Could you check a few things on this model? Use its own coordinates, in mm. A direction names the side the tool comes from. Give positions to 0.01 mm unless a question says otherwise; leave off trailing zeros. Write each loop counter-clockwise with the first axis right and the second up, starting at its lowest first coordinate (ties: lowest second). Pieces come first, ordered by that corner, then holes. Notation, with made-up numbers: M 83.25,86.5 L 106.25,86.5 A18 cw 106.25,94.5 Z; hole C 81,40 d4. An arc over 180 degrees is marked long. Answer as CSV lines item,"result". Start each with the question number.
from build123d import *

# Parameters (mm, degrees)
SKETCH1_R             = 9.525
BOSS_EXTRUDE1_DEPTH   = 3.0226
SKETCH2_W             = 5.6007
SKETCH2_H             = 19.05
CUT_EXTRUDE1_DEPTH    = 2.794
SKETCH3_W             = 19.05
SKETCH3_H             = 5.6007
CUT_EXTRUDE2_DEPTH    = 2.794
SKETCH4_W             = 3.67665
SKETCH4_H             = 19.05
CUT_EXTRUDE3_DEPTH    = 1.27
SKETCH5_W             = 19.05
SKETCH5_H             = 3.67665
CUT_EXTRUDE4_DEPTH    = 1.27
CHAMFER1_SIZE         = 1.74640875
CHAMFER1_SIZE2        = 1.008289562
CHAMFER1_PART_2_SIZE  = 1.74640875
CHAMFER1_PART_2_SIZE2 = 1.008289562
CHAMFER1_PART_3_SIZE  = 1.74640875
CHAMFER1_PART_3_SIZE2 = 1.008289562
CHAMFER1_PART_4_SIZE  = 1.74640875
CHAMFER1_PART_4_SIZE2 = 1.008289562
SKETCH6_W             = 5.880735
SKETCH6_H             = 6.905625
CUT_EXTRUDE5_DEPTH    = 2.794
SKETCH7_W             = 6.905625
SKETCH7_H             = 5.880735
CUT_EXTRUDE6_DEPTH    = 2.794


with BuildPart() as part:
    # Sketch1 → Boss-Extrude1 (new body, symmetric)
    with BuildSketch(Plane.XY):
        Circle(SKETCH1_R)
    extrude(amount=BOSS_EXTRUDE1_DEPTH, both=True)

    # Sketch2 → Cut-Extrude1 (cut)
    with BuildSketch(Plane.XY.offset(3.0226)):
        Rectangle(SKETCH2_W, SKETCH2_H)
    extrude(amount=-CUT_EXTRUDE1_DEPTH, mode=Mode.SUBTRACT)

    # Sketch3 → Cut-Extrude2 (cut)
    with BuildSketch(Plane(origin=(0, 0, -3.0226), x_dir=(-1, 0, 0), z_dir=(0, 0, -1))):
        Rectangle(SKETCH3_W, SKETCH3_H)
    extrude(amount=-CUT_EXTRUDE2_DEPTH, mode=Mode.SUBTRACT)

    # Sketch4 → Cut-Extrude3 (cut)
    with BuildSketch(Plane.XY.offset(3.0226)):
        with Locations((7.686675, 0)):
            Rectangle(SKETCH4_W, SKETCH4_H)
        with Locations((-7.686675, 0)):
            Rectangle(SKETCH4_W, SKETCH4_H)
    extrude(amount=-CUT_EXTRUDE3_DEPTH, mode=Mode.SUBTRACT)

    # Sketch5 → Cut-Extrude4 (cut)
    with BuildSketch(Plane(origin=(0, 0, -3.0226), x_dir=(-1, 0, 0), z_dir=(0, 0, -1))):
        with Locations((0, 7.686675)):
            Rectangle(SKETCH5_W, SKETCH5_H)
        with Locations((0, -7.686675)):
            Rectangle(SKETCH5_W, SKETCH5_H)
    extrude(amount=-CUT_EXTRUDE4_DEPTH, mode=Mode.SUBTRACT)

    # Chamfer1
    chamfer1_edges = [part.edges().sort_by_distance(p)[0] for p in [
        (0, 9.525, -1.7526),
    ]]
    chamfer1_side = [part.faces().sort_by_distance(p)[0] for p in [
        (0, 7.346425268, -1.7526),
    ]]
    chamfer(chamfer1_edges, length=CHAMFER1_SIZE, length2=CHAMFER1_SIZE2, reference=chamfer1_side[0])

    # Chamfer1 part 2
    chamfer1_part_2_edges = [part.edges().sort_by_distance(p)[0] for p in [
        (0, -9.525, -1.7526),
    ]]
    chamfer1_part_2_side = [part.faces().sort_by_distance(p)[0] for p in [
        (0, -7.346425268, -1.7526),
    ]]
    chamfer(chamfer1_part_2_edges, length=CHAMFER1_PART_2_SIZE, length2=CHAMFER1_PART_2_SIZE2, reference=chamfer1_part_2_side[0])

    # Chamfer1 part 3
    chamfer1_part_3_edges = [part.edges().sort_by_distance(p)[0] for p in [
        (8.556610274, -4.184500642, 1.7526),
    ]]
    chamfer1_part_3_side = [part.faces().sort_by_distance(p)[0] for p in [
        (7.346425268, 0, 1.7526),
    ]]
    chamfer(chamfer1_part_3_edges, length=CHAMFER1_PART_3_SIZE, length2=CHAMFER1_PART_3_SIZE2, reference=chamfer1_part_3_side[0])

    # Chamfer1 part 4
    chamfer1_part_4_edges = [part.edges().sort_by_distance(p)[0] for p in [
        (-9.525, 0, 1.7526),
    ]]
    chamfer1_part_4_side = [part.faces().sort_by_distance(p)[0] for p in [
        (-7.346425268, 0, 1.7526),
    ]]
    chamfer(chamfer1_part_4_edges, length=CHAMFER1_PART_4_SIZE, length2=CHAMFER1_PART_4_SIZE2, reference=chamfer1_part_4_side[0])

    # Sketch6 → Cut-Extrude5 (cut)
    with BuildSketch(Plane.XY.offset(3.0226)):
        Rectangle(SKETCH6_W, SKETCH6_H)
    extrude(amount=-CUT_EXTRUDE5_DEPTH, mode=Mode.SUBTRACT)

    # Sketch7 → Cut-Extrude6 (cut)
    with BuildSketch(Plane(origin=(0, 0, -3.0226), x_dir=(-1, 0, 0), z_dir=(0, 0, -1))):
        Rectangle(SKETCH7_W, SKETCH7_H)
    extrude(amount=-CUT_EXTRUDE6_DEPTH, mode=Mode.SUBTRACT)


solid = part.part
1. Imagine slicing it at A-A, the plane z = -0.5. Please give me the cut outline in (x, y) (3 decimals).
2. Imagine slicing it at C-C, the plane x = 0. Please give me the cut outline in (y, z) (3 decimals), plus the area to 3 significant figures.
3. Imagine slicing it at D-D, the plane z = 1. Please give me the cut outline in (x, y) (3 decimals), plus the area to 3 significant figures.
4. Imagine slicing it at B-B, the plane y = 0. Please give me the cut outline in (x, z) (3 decimals).
5. Will these pins go through, and if not, where does the flat tip stop? P1, Ø2, axis at x = -2.5, y = 7, coming from the -Z side; P2, Ø2, axis at y = 7.5, z = 1.5, coming from the +X side; P3, Ø1, axis at x = -6.5, y = -2.5, coming from the +Z side.
6. Please list where these lines run through material, in increasing order: line 1 (X direction, y = -7.25, z = 1); line 2 (Y direction, x = 3, z = -2).
7. On a 3-axis mill with a long thin cutter (end or side, diameter ignored), from which of +Z, -Z, +X, -X, +Y, -Y can I reach the whole of each face in a straight line? I mean faces 4 (the flat face through (2.94, 0, 2)), 5 (the flat face through (6, 2.8, -2)), 6 (the flat face through (-2.8, -6, 2)). Say none if no direction works.
8. Thinking about a two-plate mould opening in Y: for faces 1 (the conical face through (0.1, 8.08, -1.58)), 2 (the flat face through (0, -2.94, -2)), 3 (the flat face through (0, -4, -3.023)), which applies, pulls with the +Y half, pulls with the -Y half, needs draft (parallel to the pull), parting line crosses it, or undercut?
Solutions:
1,outline,"M -9.104,-2.8 A9.525 ccw 9.104,-2.8 L 3.453,-2.8 L 3.453,-2.94 L -3.453,-2.94 L -3.453,-2.8 Z; M -9.104,2.8 L -3.453,2.8 L -3.453,2.94 L 3.453,2.94 L 3.453,2.8 L 9.104,2.8 A9.525 ccw Z"
2,outline,"M -9.525,-0.744 L -7.779,-1.753 L -5.848,-1.753 L -5.848,-3.023 L -2.94,-3.023 L -2.94,-0.229 L 2.94,-0.229 L 2.94,-3.023 L 5.848,-3.023 L 5.848,-1.753 L 7.779,-1.753 L 9.525,-0.744 L 9.525,0.229 L -9.525,0.229 Z"
2,area,"34.4 mm²"
3,outline,"M -5.848,-7.518 A9.525 ccw -2.8,-9.104 L -2.8,-3.453 L -2.94,-3.453 L -2.94,3.453 L -2.8,3.453 L -2.8,9.104 A9.525 ccw -5.848,7.518 L -5.848,6.949 A9.082 ccw -5.848,-6.949 Z; M 2.8,-9.104 A9.525 ccw 5.848,-7.518 L 5.848,-6.949 A9.082 ccw 5.848,6.949 L 5.848,7.518 A9.525 ccw 2.8,9.104 L 2.8,3.453 L 2.94,3.453 L 2.94,-3.453 L 2.8,-3.453 Z"
3,area,"163 mm²"
4,outline,"M -9.525,-0.229 L 9.525,-0.229 L 9.525,0.744 L 7.779,1.753 L 5.848,1.753 L 5.848,3.023 L 2.94,3.023 L 2.94,0.229 L -2.94,0.229 L -2.94,3.023 L -5.848,3.023 L -5.848,1.753 L -7.779,1.753 L -9.525,0.744 Z"
5,P1,"z = -1.75"
5,P2,"x = 6.62"
5,P3,"z = 1.75"
6,line 1,"-5.85 to -2.8, 2.8 to 5.85"
6,line 2,"-5.85 to -2.94, 2.94 to 5.85"
7,face 4,"+Z"
7,face 5,"-Z, +X, -X"
7,face 6,"+Z, +Y, -Y"
8,face 1,"pulls with the +Y half"
8,face 2,"undercut"
8,face 3,"needs draft"
